Geometry: final body of the model. Coordinates: model frame, mm. Face numbers are marked on the shaded views. Give positions to 0.01 mm unless a question says otherwise; leave off trailing zeros. Loops run counter-clockwise (first coordinate to the right, second up) from the corner with the lowest first, then second, coordinate; pieces in that order, holes last.
1. Section A-A, the plane x = 10. Output: boundary loops of the cut face in (y, z), then the cut area to 3 significant figures.
2. Draft query along X for the marked faces 1 and 2. Return one class per face: +X half, -X half, draft (parallel to the pull), parting line (faces both ways), or undercut.
3. Section C-C, the plane z = 2.1. Output: boundary loops of the cut face in (x, y).
4. Material intervals for line 1 along Y through (x, z) = (10, 3.9); line 2 along Y through (x, z) = (12, 0.5); line 3 along X through (y, z) = (13, 1.1), sorted ascending.
5. First-contact query: P1, Ø6, axis at x = 10, y = 98.4, coming from the +Z side. Flat tip, straight axial feed; report the tip coordinate or a pass-through.
6. Section B-B, the plane y = 98.4. Output: boundary loops of the cut face in (x, z).
Autodesk Inventor part; units mm, degrees
ref_plane "YZ Plane" through (0, 0, 0) normal (1, 0, 0) x (0, 1, 0)
ref_plane "XZ Plane" through (0, 0, 0) normal (0, 1, 0) x (-1, 0, 0)
ref_plane "XY Plane" through (0, 0, 0) normal (0, 0, 1) x (1, 0, 0)
sketch "スケッチ1" plane through (0, 0, 0) normal (0, 0, 1) x (1, 0, 0)
  line L0 (0, 0) -> (20, 0)
  line L1 (20, 0) -> (20, 108.4)
  line L2 (20, 108.4) -> (0, 108.4)
  line L3 (0, 108.4) -> (0, 0)
  circle A0 centre (10, 98.4) radius 5
  circle A1 centre (10, 10) radius 5
  dimension "d0" = 20
  dimension "d1" = 108.4
  dimension "d2" = 10
  dimension "d3" = 10
  dimension "d4" = 10
  dimension "d5" = 10
  dimension "d6" = 10
  dimension "d7" = 10
extrude "押し出し1" add sketch "スケッチ1" along normal blind 5
properties part number "rocker_bogie_plate" material "アルミニウム 6061"
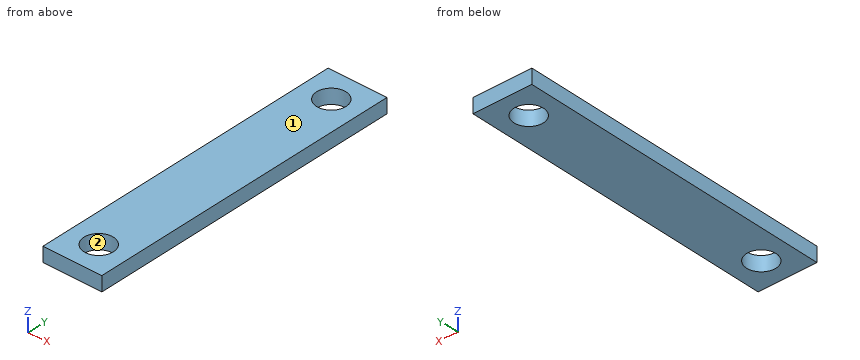
Answers below:
1. outline: (0, 0) - (5, 0) - (5, 5) - (0, 5) - close; (15, 0) - (93.4, 0) - (93.4, 5) - (15, 5) - close; (103.4, 0) - (108.4, 0) - (108.4, 5) - (103.4, 5) - close
1. area: 442 mm2
2. face 1: draft
2. face 2: undercut
3. outline: (0, 0) - (20, 0) - (20, 108.4) - (0, 108.4) - close; hole circle Ø10 at (10, 10); hole circle Ø10 at (10, 98.4)
4. line 1: y = 0 to 5, 15 to 93.4, 103.4 to 108.4
4. line 2: y = 0 to 5.42, 14.58 to 93.82, 102.98 to 108.4
4. line 3: x = 0 to 6, 14 to 20
5. P1: passes through
6. outline: (0, 0) - (5, 0) - (5, 5) - (0, 5) - close; (15, 0) - (20, 0) - (20, 5) - (15, 5) - close
